from build123d import *

# Parameters (mm, degrees)
SKETCH1_W                  = 10
SKETCH1_H                  = 60
SKETCH2_R                  = 30
BOSS_EXTRUDE1_DEPTH        = 45
CUT_EXTRUDE1_DEPTH         = 102.118742081
SKETCH4_W                  = 55
SKETCH4_H                  = 15
F_12_0_12_DIAMETER_HOLE1_D = 12


with BuildPart() as part:
    # Sketch1 → Revolve1 (revolve)
    with BuildSketch(Plane(origin=(0, 0, 0), x_dir=(-1, 0, 0), z_dir=(0, 0, -1)), mode=Mode.PRIVATE) as revolve1_sk:
        with Locations((-5, 30)):
            Rectangle(SKETCH1_W, SKETCH1_H)
    revolve(revolve1_sk.sketch.rotate(Axis((10, 0, 0), (-1, 0, 0)), 270), axis=Axis((10, 0, 0), (-1, 0, 0)))

    # Sketch2 → Boss-Extrude1 (add)
    with BuildSketch(Plane.ZY):
        with Locations(Location((0, 0, 0), (0, 0, 180))):
            Circle(SKETCH2_R)
    extrude(amount=BOSS_EXTRUDE1_DEPTH)

    # Sketch3 → Cut-Extrude1 (cut, through all)
    with BuildSketch(Plane.ZY.offset(45)):
        with BuildLine():
            Line((-7.5, 22.495647676), (-7.5, 12.990381057))
            ThreePointArc((-7.5, 12.990381057), (0, 15), (7.5, 12.990381057))
            Line((7.5, 12.990381057), (7.5, 22.495647676))
            Line((7.5, 22.495647676), (-7.5, 22.495647676))
        make_face()
    extrude(amount=-CUT_EXTRUDE1_DEPTH, mode=Mode.SUBTRACT)

    # Sketch4 → Cut-Revolve1 (revolve, cut)
    with BuildSketch(Plane(origin=(0, 0, 0), x_dir=(-1, 0, 0), z_dir=(0, 0, -1))):
        with Locations((17.5, 7.5)):
            Rectangle(SKETCH4_W, SKETCH4_H)
    revolve(axis=Axis((10, 0, 0), (-1, 0, 0)), mode=Mode.SUBTRACT)

    # Ø12.0 (12) Diameter Hole1 (through all)
    with Locations(Plane.ZY):
        with Locations((-38.97114317, 22.5), (38.97114317, 22.5), (0, -45)):
            Hole(F_12_0_12_DIAMETER_HOLE1_D / 2)


solid = part.part
Model file for the job. Use its own axes, mm. A direction names the side the tool comes from. Give positions to 0.01 mm unless a question says otherwise; leave off trailing zeros. Order: outer loops, then holes, each group sorted by start corner. A loop starts at its lowest first (then second) coordinate and runs counter-clockwise, first axis right, second up. Notation, with made-up numbers: (65.25, -38.75) - (81.25, -38.75) arc R19 ccw to (81.25, -27.75) - close; hole circle Ø5 at (67.25, 14.25). An arc over 180 degrees is marked (long way). Return JSON: item names as keys, results as strings.
1) Cut at C-C, the plane x = -40.5. Give the cut face in (y, z).
Geometry says:
{"outline": "circle Ø60 at (0, 0); hole (12.99, -7.5) - (22.5, -7.5) - (22.5, 7.5) - (12.99, 7.5) arc R15 ccw (long way) to start"}
2) 3-axis set-ups, long thin cutter, end or side, ignore diameter. For faces 1 (the flat face through (-18, 22.496, 0)), 2 (the cylindrical face through (-22.185, -25.296, -16.128)), 3 (the flat face through (10, -12, -12)): which of +Z, -Z, +X, -X, +Y, -Y reach the whole face in a straight line?
Geometry says:
{"face 1": "+X, -X", "face 2": "-X", "face 3": "+Z, -Z, +X, +Y, -Y"}
3) Cut at B-B, the plane z = 0. Give the cut face in (x, y).
Geometry says:
{"outline": "(-45, -30) - (0, -30) - (0, -39) - (10, -39) - (10, -15) - (-45, -15) - close; (-45, 22.5) - (10, 22.5) - (10, 60) - (0, 60) - (0, 30) - (-45, 30) - close; (0, -60) - (10, -60) - (10, -51) - (0, -51) - close"}
4) Probe line 1 (Y direction, x = -33, z = 0); line 2 (X direction, y = -21.5, z = 55); line 3 (Z direction, x = -26.5, y = 11.5). List the from-to ranges inside material, lowest first. Write a range as from..to.
Geometry says:
{"line 1": "-30..-15, 22.5..30", "line 2": "0..10", "line 3": "-27.71..-9.63, 9.63..27.71"}
5) Pull direction Y, two halves, no side cores. Call faces 4 (the cylindrical face through (4.93, 2.64, -59.94)), 5 (the flat face through (-45, -14, -6)), 6 (the flat face through (-18, 18, 7.5)): pulls with the +Y half, pulls with the -Y half, needs draft (parallel to the pull), parting line crosses it, or undercut.
Geometry says:
{"face 4": "parting line crosses it", "face 5": "needs draft", "face 6": "undercut"}
6) Cut at A-A, the plane y = 0. Give the cut face in (x, z), plus the area to 3 significant figures.
Geometry says:
{"outline": "(-45, -30) - (0, -30) - (0, -60) - (10, -60) - (10, -15) - (-45, -15) - close; (-45, 15) - (10, 15) - (10, 60) - (0, 60) - (0, 30) - (-45, 30) - close", "area": "2,250 mm²"}
7) Flat gauge pins, fed straight in: P1, Ø7.5, axis at x = -19.5, y = 16.5, coming from the +Z side; P2, Ø3, axis at x = -28.5, z = -23, coming from the -Y side; P3, Ø10, axis at x = 0, z = -37.5, coming from the +Y side; P4, Ø11, axis at y = 22.5, z = -38.97, coming from the -X side. Where does each tip first touch, or does it go through?
Geometry says:
{"P1": "z = 27.16", "P2": "y = -20.92", "P3": "y = 50.44", "P4": "through"}
8) Cut at D-D, the plane z = 39.5. Give the cut face in (x, y), plus the area to 3 significant figures.
Geometry says:
{"outline": "(0, -45.16) - (10, -45.16) - (10, 16.52) - (0, 16.52) - close; (0, 28.48) - (10, 28.48) - (10, 45.16) - (0, 45.16) - close", "area": "784 mm²"}
